```python
from build123d import *

# Parameters (mm, degrees)
SKETCH_10_R         = 1.65
EXTRUDE_1_DEPTH     = 3
EXTRUDE_START       = 3
EXTRUDE_2_DEPTH     = 7
EXTRUDE_3_DEPTH     = 13
CHAMFER_1_SIZE      = 7
EXTRUDE_5_DEPTH     = 10
EXTRUDE_START_2     = -1.1
SKETCH_16_R         = 1.65
EXTRUDE_6_DEPTH     = 4.1
EXTRUDE_7_DEPTH     = 16
SKETCH_18_W         = 21
SKETCH_18_H         = 15.2
CUT_EXTRUDE_1_DEPTH = 14.1
FILLET_1_R          = 1


with BuildPart() as part:
    # 草图10 → 凸台-拉伸1 (new body)
    with BuildSketch(Plane.XY):
        Polygon((-92.4, -8), (-21.435028843, -8), (13.564971157, 27), (92.4, 27), (92.4, 8), (21.435028843, 8), (-13.564971157, -27), (-92.4, -27), align=None)
        with Locations((-82.4, -17.5)):
            Circle(SKETCH_10_R, mode=Mode.SUBTRACT)
        with Locations((82.4, 17.5)):
            Circle(SKETCH_10_R, mode=Mode.SUBTRACT)
    extrude(amount=EXTRUDE_1_DEPTH)

    # 草图11 → 凸台-拉伸2 (add)
    with BuildSketch(Plane.XY.offset(EXTRUDE_START)):
        Polygon((-73.4, -8), (-73.4, -27), (-13.564971157, -27), (21.435028843, 8), (71.4, 8), (71.4, 27), (13.564971157, 27), (-21.435028843, -8), align=None)
    extrude(amount=EXTRUDE_2_DEPTH)

    # 草图12 → 凸台-拉伸3 (add)
    with BuildSketch(Plane.XY.offset(EXTRUDE_START)):
        Polygon((-92.4, -8), (-21.435028843, -8), (13.564971157, 27), (92.4, 27), (92.4, 24), (14.807611845, 24), (-20.192388155, -11), (-92.4, -11), align=None)
        Polygon((-92.4, -24), (-92.4, -27), (-13.564971157, -27), (21.435028843, 8), (92.4, 8), (92.4, 11), (20.192388155, 11), (-14.807611845, -24), align=None)
    extrude(amount=EXTRUDE_3_DEPTH)

    # 倒角1
    chamfer_1_edges = [part.edges().sort_by_distance(p)[0] for p in [
        (71.4, 17.5, 10),
        (-73.4, -17.5, 10),
    ]]
    chamfer(chamfer_1_edges, length=CHAMFER_1_SIZE - 0.0001)  # a hair under: the kernel refuses the full size

    # 草图15 → 凸台-拉伸5 (add)
    with BuildSketch(Plane.XY.offset(3)):
        Polygon((-69.4, -11), (-69.4, -15), (-18.535533906, -15), (16.464466094, 20), (67.4, 20), (67.4, 24), (14.807611845, 24), (-20.192388155, -11), align=None)
        Polygon((-69.4, -20), (-69.4, -24), (-14.807611845, -24), (20.192388155, 11), (67.4, 11), (67.4, 15), (18.535533906, 15), (-16.464466094, -20), align=None)
    extrude(amount=EXTRUDE_5_DEPTH)

    # 草图16 → 凸台-拉伸6 (add)
    with BuildSketch(Plane.XY.offset(EXTRUDE_START_2)):
        Polygon((-92.4, -8), (-92.4, -27), (-13.564971157, -27), (20.335028843, 6.9), (92.4, 6.9), (92.4, 28.1), (14.664971157, 28.1), (-21.435028843, -8), align=None)
        with Locations((-82.4, -17.5)):
            Circle(SKETCH_16_R, mode=Mode.SUBTRACT)
        with Locations((82.4, 17.5)):
            Circle(SKETCH_16_R, mode=Mode.SUBTRACT)
    extrude(amount=EXTRUDE_6_DEPTH)

    # 草图17 → 凸台-拉伸7 (add)
    with BuildSketch(Plane.XY):
        Polygon((92.4, 28.1), (92.4, 24), (14.807611845, 24), (12.686291501, 26.121320344), (14.664971157, 28.1), align=None)
        Polygon((92.4, 6.9), (20.335028843, 6.9), (18.213708499, 9.021320344), (20.192388155, 11), (92.4, 11), align=None)
    extrude(amount=EXTRUDE_7_DEPTH)

    # 草图18 → 切除-拉伸1 (cut)
    with BuildSketch(Plane.XY.offset(16)):
        with Locations((81.9, 17.5)):
            Rectangle(SKETCH_18_W, SKETCH_18_H)
    extrude(amount=-CUT_EXTRUDE_1_DEPTH, mode=Mode.SUBTRACT)


with BuildPart() as cut_extrude_1_kept_piece:
    # of the separate pieces the step leaves, the one the design keeps (cut_extrude_1_pieces_kept)
    add(part.part.solids().sort_by_distance((-73.4, -24, 3.0001))[0])

    # 圆角1
    fillet_1_edges = [cut_extrude_1_kept_piece.edges().sort_by_distance(p)[0] for p in [
        (-21.435028843, -8, 7.45),
        (-13.564971157, -27, 7.45),
        (-18.535533906, -15, 11.5),
        (16.464466094, 20, 11.5),
        (-16.464466094, -20, 11.5),
        (18.535533906, 15, 11.5),
        (20.335028843, 6.9, 7.45),
        (14.664971157, 28.1, 7.45),
        (14.807611845, 24, 14.5),
        (-20.192388155, -11, 14.5),
        (-14.807611845, -24, 14.5),
        (20.192388155, 11, 14.5),
    ]]
    fillet(fillet_1_edges, radius=FILLET_1_R)


solid = cut_extrude_1_kept_piece.part
```
CAD build for the part. Positions are in the model's coordinates, mm. A direction names the side the tool comes from. Round coordinates to 2 decimals unless told otherwise and drop trailing zeros. Loops run counter-clockwise (first coordinate to the right, second up) from the corner with the lowest first, then second, coordinate; pieces in that order, holes last. Notation, with made-up numbers: M 73.5,49.25 L 129.5,49.25 A20 cw 129.5,72.25 Z; hole C 10,67 d11. An arc over 180 degrees is marked long. Return JSON: item names as keys, results as strings. Group by question number.
(1) Saw through at B-B, the plane y = 17.5. List the corners of the cut face in (x, z), and give its area (3 significant figures).
(2) Saw through at D-D, the plane z = 4.75. List the corners of the cut face in (x, y), and give its area (3 significant figures).
(3) Drop flat-ended pins along their axis: P1, Ø6.5, axis at x = -85.5, y = -20, coming from the +Z side; P2, Ø4.5, axis at y = 12.5, z = 11.5, coming from the +X side; P3, Ø5, axis at x = 67, z = 9, coming from the -Y side. Give the stop position or say it passes through.
(4) Mould opens along X. For faces 4 (the flat face through (44, 15, 11)), 5 (the flat face through (-1.276, 2.259, 11.479)), 6 (the flat face through (3.152, -10.283, 7.33)), 7 (the flat face through (-1, -6, 13)) say: +X half, -X half, draft (parallel to the pull), parting line (faces both ways), or undercut.
(5) Saw through at A-A, the plane x = -82.4. List the corners of the cut face in (y, z).
(6) Saw through at C-C, the plane x = 57. List the corners of the cut face in (y, z).
(7) Wall check: probe 1 along Y at (x, z) = (-84, 5.75); probe 2 along Y at (x, z) = (-82.4, 1.5); probe 3 along Z at (x, y) = (-14, -23). Give the ranges that are in metal, low to high. Write a range as [from, to].
(8) Tool access for faces 1 (the flat face through (47.6, 24, 13.3)), 2 (the flat face through (-43, -20, 12)), 3 (the flat face through (-57, -8, 7)): list every direction of +Z, -Z, +X, -X, +Y, -Y with a clear straight run to the whole face (end or side of a thin tool).
Answer list:
{
 "1": {"outline": "M 4.06,-1.1 L 80.75,-1.1 L 80.75,1.9 L 71.4,1.9 L 71.4,3 L 64.4,10 L 13.96,10 L 13.96,13 L 8.31,13 L 8.31,16 L 4.06,16 Z; M 84.05,-1.1 L 92.4,-1.1 L 92.4,1.9 L 84.05,1.9 Z", "area": "818 mm2"},
 "2": {"outline": "M -92.4,-27 L -13.98,-27 A1 ccw -13.27,-26.71 L 20.04,6.61 A1 cw 20.75,6.9 L 92.4,6.9 L 92.4,9.9 L 71.4,9.9 L 71.4,11 L 69.65,11 L 69.65,24 L 71.4,24 L 71.4,25.1 L 92.4,25.1 L 92.4,28.1 L 15.08,28.1 A1 ccw 14.37,27.81 L -21.14,-7.71 A1 cw -21.85,-8 L -92.4,-8 L -92.4,-11 L -71.65,-11 L -71.65,-24 L -92.4,-24 Z", "area": "3,340 mm2"},
 "3": {"P1": "z = 3", "P2": "x = 71.4", "P3": "y = 6.9"},
 "4": {"face 4": "draft", "face 5": "undercut", "face 6": "+X half", "face 7": "undercut"},
 "5": {"outline": "M -27,-1.1 L -19.15,-1.1 L -19.15,3 L -24,3 L -24,16 L -27,16 Z; M -15.85,-1.1 L -8,-1.1 L -8,16 L -11,16 L -11,3 L -15.85,3 Z"},
 "6": {"outline": "M 6.9,-1.1 L 28.1,-1.1 L 28.1,16 L 24,16 L 24,13 L 20,13 L 20,10 L 15,10 L 15,13 L 11,13 L 11,16 L 6.9,16 Z"},
 "7": {"probe 1": "[-27, -24], [-11, -8]", "probe 2": "[-27, -19.15], [-15.85, -8]", "probe 3": "[-1.1, 13]"},
 "8": {"face 1": "+Z, +X", "face 2": "+Z, -X", "face 3": "+Z, -Z, -X, +Y"}
}
